Part model, mm, in its own coordinate system. A direction names the side the tool comes from. Coordinates: 2 decimals unless noted, no trailing zeros. Write each loop counter-clockwise with the first axis right and the second up, starting at its lowest first coordinate (ties: lowest second). Pieces come first, ordered by that corner, then holes. Notation, with made-up numbers: (49, 88) - (108, 88) arc R12 ccw to (108, 94) - close; hole circle Ø11 at (2.5, -38.75). An arc over 180 degrees is marked (long way). Use one line per item in the form item = value. Start each with the question number.
Autodesk Inventor part; units mm, degrees
ref_plane "YZ Plane" through (0, 0, 0) normal (1, 0, 0) x (0, 1, 0)
ref_plane "XZ Plane" through (0, 0, 0) normal (0, 1, 0) x (-1, 0, 0)
ref_plane "XY Plane" through (0, 0, 0) normal (0, 0, 1) x (1, 0, 0)
sketch "Sketch1" plane through (0, 0, 0) normal (0, 0, 1) x (1, 0, 0)
  circle A0 centre (0, 0) radius 17.399
  dimension "d0" = 34.798
extrude "Extrusion1" add sketch "Sketch1" along normal blind 30.734
sketch "Sketch2" plane through (0, 0, 30.734) normal (0, 0, 1) x (1, 0, 0)
  circle A0 centre (0, 0) radius 18.415
  dimension "d3" = 36.83
extrude "Extrusion2" add sketch "Sketch2" along normal blind 23.876
sketch "Sketch3" plane through (0, 0, 54.61) normal (0, 0, 1) x (1, 0, 0)
  line L0 (0, 0) -> (0, -7.112) construction
  circle A0 centre (0, -7.112) radius 5.969
  dimension "d6" = 7.112
  dimension "d7" = 11.938
extrude "Extrusion3" add sketch "Sketch3" along normal blind 6.096
sketch "Sketch4" plane through (0, -7.112, 60.706) normal (0, 0, 1) x (1, 0, 0)
  circle A0 centre (0, 0) radius 3.048
  point P0 (0, 7.112)
  dimension "d10" = 6.096
extrude "Extrusion4" add sketch "Sketch4" along normal blind 16.002
properties part number "Drivetrain_Motor"
Q1. Slice it at D-D (y = 8). List the corners of the cut face in (x, z).
Q2. Which spindle directions (+Z, -Z, +X, -X, +Y, -Y) get a long thin tool onto all of the face, cutting with end or side? Do faces 1 (the cylindrical face through (-0.78, -13.03, 57.62)), 2 (the cylindrical face through (-3.772, 16.985, 15.152)), 3 (the cylindrical face through (-14.61, 11.21, 42.5)). Say none if no direction does.
Q3. Slice it at A-A (y = 0). List the corners of the cut face in (x, z) (3 decimals).
Q4. Drill centre lines: probe 1 along Z at (x, y) = (-10, 14.5); probe 2 along Z at (x, y) = (-3, 4.5); probe 3 along Y at (x, z) = (0.5, 17). Where is each one in solid material? Low to high.
Q5. Slice it at B-B (x = 0). List the corners of the cut face in (y, z) (3 decimals).
Q6. Pin check, flat tips, straight feed: P1, Ø3, axis at y = 1, z = 61, coming from the -X side; P2, Ø6, axis at y = -4.5, z = 8, coming from the -X side; P3, Ø6, axis at x = 9.5, z = 47, coming from the -Y side; P4, Ø12, axis at y = 7, z = 9, coming from the -X side. Stop position of each tip, or through.
Q7. Slice it at C-C (z = 12.5). List the corners of the cut face in (x, y).
Solution:
q1.outline = (-16.59, 30.73) - (-15.45, 30.73) - (-15.45, 0) - (15.45, 0) - (15.45, 30.73) - (16.59, 30.73) - (16.59, 54.61) - (-16.59, 54.61) - close
q2.face_1 = +Z
q2.face_2 = -Z
q2.face_3 = +Z, -Z
q3.outline = (-18.415, 30.734) - (-17.399, 30.734) - (-17.399, 0) - (17.399, 0) - (17.399, 30.734) - (18.415, 30.734) - (18.415, 54.61) - (-18.415, 54.61) - close
q4.probe_1 = 30.73 to 54.61
q4.probe_2 = 0 to 54.61
q4.probe_3 = -17.39 to 17.39
q5.outline = (-18.415, 30.734) - (-17.399, 30.734) - (-17.399, 0) - (17.399, 0) - (17.399, 30.734) - (18.415, 30.734) - (18.415, 54.61) - (-1.143, 54.61) - (-1.143, 60.706) - (-4.064, 60.706) - (-4.064, 76.708) - (-10.16, 76.708) - (-10.16, 60.706) - (-13.081, 60.706) - (-13.081, 54.61) - (-18.415, 54.61) - close
q6.P1 = through
q6.P2 = -17.33
q6.P3 = -17.23
q6.P4 = -17.37
q7.outline = circle Ø34.8 at (0, 0)
